For this review, take the finished solid that the model builds, in its own axes (mm). A direction names the side the tool comes from. Give positions to 0.01 mm unless a question says otherwise; leave off trailing zeros. Write each loop counter-clockwise with the first axis right and the second up, starting at its lowest first coordinate (ties: lowest second). Pieces come first, ordered by that corner, then holes.
Q1. We need section A-A (z = 1.55). Write out the cut boundary in (x, y), then the cut area to 3 significant figures.
Q2. We need section C-C (x = -18). Write out the cut boundary in (y, z) (3 decimals).
Q3. Insertion check: P1, Ø10, axis at x = 2, y = -0.5, coming from the +Z side; P2, Ø1, axis at x = 5, z = 1.5, coming from the -Y side. Each pin has a flat end and moves straight along its axis. Give the tip position at first contact, or say it passes through.
Q4. We need section B-B (y = -2.5). Write out the cut boundary in (x, z) (3 decimals).
Q5. Mouldability with a two-part tool opening along Y and no side actions: class faces 1 (the flat face through (7, -7, 0)), 2 (the flat face through (12.219, 12.566, 1.565)), 3 (the flat face through (-12.219, -12.566, 1.565)), 4 (the cylindrical face through (-0.4, 16.19, 1.57)) as released by +Y, released by -Y, zero draft, split by the parting line, or undercut.
Q6. Machinability: for faces 5 (the cylindrical face through (11.4, 0.1, 1.6)), 6 (the flat face through (7, -7, 3.175)), which of the approach directions +Z, -Z, +X, -X, +Y, -Y give a long, thin tool a straight path to every point of the face, cutting with its end or side? Answer none if there is none.
Q7. For line 1 (Y direction, x = 0.5, z = 1); line 2 (Y direction, x = 19, z = 2.75); line 3 (Y direction, x = 16.5, z = 2.2), list the stretches that pass through material, from the lowest coordinate up.
Q8. We need section D-D (y = -15). Write out the cut boundary in (x, z) (3 decimals), then the cut area to 3 significant figures.
```python
from build123d import *

# Parameters (mm, degrees)
SKETCH2_R           = 1.8542
BOSS_EXTRUDE1_DEPTH = 3.175
FILLET1_R           = 5


with BuildPart() as part:
    # Sketch2 → Boss-Extrude1 (new body)
    with BuildSketch(Plane.XY):
        Polygon((0, 24.784092681), (24.784092681, 0), (0, -24.784092681), (-24.784092681, 0), align=None)
        with Locations((0, 18)):
            Circle(SKETCH2_R, mode=Mode.SUBTRACT)
        with Locations((-18, 0)):
            Circle(SKETCH2_R, mode=Mode.SUBTRACT)
        with Locations((0, -18)):
            Circle(SKETCH2_R, mode=Mode.SUBTRACT)
        with Locations((18, 0)):
            Circle(SKETCH2_R, mode=Mode.SUBTRACT)
        Polygon((0, 13.470384182), (13.470384182, 0), (0, -13.470384182), (-13.470384182, 0), align=None, mode=Mode.SUBTRACT)
    extrude(amount=BOSS_EXTRUDE1_DEPTH)

    # Fillet1
    fillet1_edges = [part.edges().sort_by_distance(p)[0] for p in [
        (0, 13.470384182, 1.5875),
        (-13.470384182, 0, 1.5875),
        (0, -13.470384182, 1.5875),
        (13.470384182, 0, 1.5875),
    ]]
    fillet(fillet1_edges, radius=FILLET1_R)


solid = part.part
```
Computed:
1. outline: (-24.78, 0) - (0, -24.78) - (24.78, 0) - (0, 24.78) - close; hole circle Ø3.71 at (-18, 0); hole (-9.93, -3.54) - (-3.54, -9.93) arc R5 ccw to (3.54, -9.93) - (9.93, -3.54) arc R5 ccw to (9.93, 3.54) - (3.54, 9.93) arc R5 ccw to (-3.54, 9.93) - (-9.93, 3.54) arc R5 ccw to start; hole circle Ø3.71 at (0, -18); hole circle Ø3.71 at (0, 18); hole circle Ø3.71 at (18, 0)
1. area: 844 mm2
2. outline: (-6.784, 0) - (-1.854, 0) - (-1.854, 3.175) - (-6.784, 3.175) - close; (1.854, 0) - (6.784, 0) - (6.784, 3.175) - (1.854, 3.175) - close
3. P1: passes through
3. P2: stops at y = -20.28
4. outline: (-22.284, 0) - (-10.729, 0) - (-10.729, 3.175) - (-22.284, 3.175) - close; (10.729, 0) - (22.284, 0) - (22.284, 3.175) - (10.729, 3.175) - close
5. face 1: zero draft
5. face 2: released by +Y
5. face 3: released by -Y
5. face 4: undercut
6. face 5: +Z, -Z
6. face 6: +Z, +X, -X, +Y, -Y
7. line 1: y = -24.28 to -19.79, -16.21 to -11.37, 11.37 to 16.21, 19.79 to 24.28
7. line 2: y = -5.78 to -1.56, 1.56 to 5.78
7. line 3: y = -8.28 to -1.09, 1.09 to 8.28
8. outline: (-9.784, 0) - (9.784, 0) - (9.784, 3.175) - (-9.784, 3.175) - close
8. area: 62.1 mm2
